```python
from build123d import *

# Parameters (mm, degrees)
SKETCH1_R                           = 37.5
BOSS_EXTRUDE1_DEPTH                 = 10
M2X0_4_TAPPED_HOLE2_D               = 1.6
M2X0_4_TAPPED_HOLE2_CSINK_D         = 2.05
M2X0_4_TAPPED_HOLE2_CSINK_ANGLE     = 90
M2X0_4_TAPPED_HOLE1_D               = 1.6
M2X0_4_TAPPED_HOLE1_DEPTH           = 6
M2X0_4_TAPPED_HOLE1_TIP             = 0.480688495
M2X0_4_TAPPED_HOLE1_ON_FACE_2_D     = 1.6
M2X0_4_TAPPED_HOLE1_ON_FACE_2_DEPTH = 6
M2X0_4_TAPPED_HOLE1_ON_FACE_2_TIP   = 0.480688495
CHAMFER1_SIZE                       = 0.2
SKETCH11_R                          = 19.5
BOSS_EXTRUDE2_DEPTH                 = 10
SKETCH12_R                          = 8
CUT_EXTRUDE1_DEPTH                  = 106.913751518
M3_CLEARANCE_HOLE1_D                = 3.4


with BuildPart() as part:
    # Sketch1 → Boss-Extrude1 (new body)
    with BuildSketch(Plane(origin=(0, 0, 0), x_dir=(1, 0, 0), z_dir=(0, 1, 0))):
        with BuildLine():
            Line((-55.5, 55.5), (63.5, 55.5))
            Line((63.5, 55.5), (63.5, 0))
            ThreePointArc((63.5, 0), (44.901280605, -44.901280605), (0, -63.5))
            Line((0, -63.5), (-55.5, -63.5))
            Line((-55.5, -63.5), (-55.5, 55.5))
        make_face()
        with Locations(Location((0, 0, 0), (0, 0, 270))):
            Circle(SKETCH1_R, mode=Mode.SUBTRACT)
    extrude(amount=BOSS_EXTRUDE1_DEPTH)

    # M2x0.4 Tapped Hole2 (through all)
    with Locations(Plane(origin=(0, 10, 0), x_dir=(1, 0, 0), z_dir=(0, 1, 0))):
        with Locations((37.476659403, 37.476659403), (-37.476659403, 37.476659403), (-37.476659403, -37.476659403), (37.476659403, -37.476659403)):
            CounterSinkHole(M2X0_4_TAPPED_HOLE2_D / 2, M2X0_4_TAPPED_HOLE2_CSINK_D / 2, counter_sink_angle=M2X0_4_TAPPED_HOLE2_CSINK_ANGLE)

    # M2x0.4 Tapped Hole1
    with Locations(Plane(origin=(63.5, 5, -50.5), x_dir=(0, 0, 1), z_dir=(1, 0, 0))):
        with Locations((0, 0), (40, 0)):
            Hole(M2X0_4_TAPPED_HOLE1_D / 2, depth=M2X0_4_TAPPED_HOLE1_DEPTH)
            with Locations((0, 0, -(M2X0_4_TAPPED_HOLE1_DEPTH + M2X0_4_TAPPED_HOLE1_TIP / 2))):  # 118° drill point
                Cone(0, M2X0_4_TAPPED_HOLE1_D / 2, M2X0_4_TAPPED_HOLE1_TIP, mode=Mode.SUBTRACT)

    # M2x0.4 Tapped Hole1 on face 2
    with Locations(Plane(origin=(-50.5, 5, 63.5), x_dir=(1, 0, 0), z_dir=(0, 0, 1))):
        with Locations((0, 0), (40, 0)):
            Hole(M2X0_4_TAPPED_HOLE1_ON_FACE_2_D / 2, depth=M2X0_4_TAPPED_HOLE1_ON_FACE_2_DEPTH)
            with Locations((0, 0, -(M2X0_4_TAPPED_HOLE1_ON_FACE_2_DEPTH + M2X0_4_TAPPED_HOLE1_ON_FACE_2_TIP / 2))):  # 118° drill point
                Cone(0, M2X0_4_TAPPED_HOLE1_ON_FACE_2_D / 2, M2X0_4_TAPPED_HOLE1_ON_FACE_2_TIP, mode=Mode.SUBTRACT)

    # Chamfer1
    chamfer1_edges = [part.edges().sort_by_distance(p)[0] for p in [
        (-9.7, 5, 63.5),
        (-49.7, 5, 63.5),
        (63.5, 5, -9.7),
        (63.5, 5, -49.7),
    ]]
    chamfer(chamfer1_edges, length=CHAMFER1_SIZE)

    # Sketch11 → Boss-Extrude2 (add, through all)
    with BuildSketch(Plane(origin=(0, 10, 0), x_dir=(1, 0, 0), z_dir=(0, 1, 0))):
        with Locations((-14.752685571, 55.057772098)):
            Circle(SKETCH11_R)
        with Locations((-55.057772098, 14.752685571)):
            Circle(SKETCH11_R)
    extrude(amount=-BOSS_EXTRUDE2_DEPTH)

    # Sketch12 → Cut-Extrude1 (cut, through all)
    with BuildSketch(Plane(origin=(0, 10, 0), x_dir=(1, 0, 0), z_dir=(0, 1, 0))):
        with Locations(Location((-14.752685571, 55.057772098, 0), (0, 0, 270))):
            Circle(SKETCH12_R)
        with Locations(Location((-55.057772098, 14.752685571, 0), (0, 0, 270))):
            Circle(SKETCH12_R)
    extrude(amount=-CUT_EXTRUDE1_DEPTH, mode=Mode.SUBTRACT)

    # M3 Clearance Hole1 (through all)
    with Locations(Plane(origin=(1225.129186233, 0, -788.179357161), x_dir=(0.12314040674573719, 0, 0.992389258419545), z_dir=(0, -1, 0))):
        with Locations((602.6321738, 1378.806890422), (624.895157282, 1365.414371373), (602.165403824, 1352.830321638), (587.985457399, 1327.987745968), (574.59293835, 1305.724762486), (562.008888615, 1328.454515944)):
            Hole(M3_CLEARANCE_HOLE1_D / 2)


solid = part.part
```
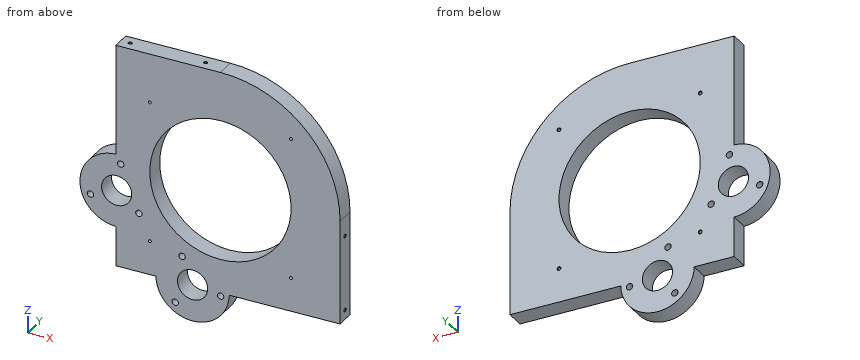
The model under review builds one solid part; all positions refer to its coordinate system, in mm. Coordinates: 2 decimals unless noted, no trailing zeros. Order: outer loops, then holes, each group sorted by start corner. A loop starts at its lowest first (then second) coordinate and runs counter-clockwise, first axis right, second up. Notation, with made-up numbers: M -11.5,75 L 40.5,75 A23 cw 40.5,99 Z; hole C -18,12.5 d9. An arc over 180 degrees is marked long. One line per question, with ' | ' between items.
(1) Add section C-C, the plane x = 49. Write out the cut boundary in (y, z), then the cut area to 3 significant figures.
Geometry results:
outline: M 0,-55.5 L 10,-55.5 L 10,40.39 L 0,40.39 Z | area: 959 mm²
(2) Add section B-B, the plane z = 20. Write out the cut boundary in (x, y), then the cut area to 3 significant figures.
Geometry results:
outline: M -55.5,0 L -31.72,0 L -31.72,10 L -55.5,10 Z; M 31.72,0 L 60.27,0 L 60.27,10 L 31.72,10 Z | area: 523 mm²
(3) Insertion check: pin 1 (4.5 mm diameter, centred on x = -52.94, z = 0.1, fed in from +Y); pin 2 (1 mm diameter, centred on x = 25, y = 6.5, fed in from -Z); pin 3 (1.8 mm diameter, centred on y = 5, z = -50.5, fed in from +X); pin 4 (1.3 mm diameter, centred on x = -10.5, y = 5, fed in from +Z). Each pin has a flat end and moves straight along its axis. Give the tip position at first contact, or say it passes through.
Geometry results:
pin 1: stops at y = 10 | pin 2: stops at z = -55.5 | pin 3: stops at x = 63.4 | pin 4: stops at z = 57.41
(4) For probe 1 along Z at (x, y) = (-14.5, 5); probe 2 along Y at (x, z) = (60.5, -10.5); probe 3 along X at (y, z) = (5.5, 38), list the stretches that pass through material, from the lowest coordinate up. Write a range as from..to.
Geometry results:
probe 1: z = -74.56..-63.05, -47.06..-34.58, 34.58..63.5 | probe 2: y = 0..4.2, 5.8..10 | probe 3: x = -55.5..-38.08, -36.87..36.87, 38.08..50.87
(5) Add section A-A, the plane x = 32.5. Write out the cut boundary in (y, z).
Geometry results:
outline: M 0,-55.5 L 10,-55.5 L 10,-18.71 L 0,-18.71 Z; M 0,18.71 L 10,18.71 L 10,54.55 L 0,54.55 Z
